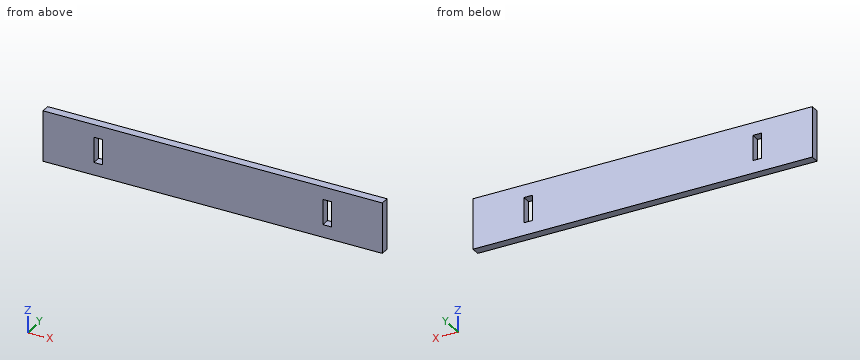
```python
from build123d import *

# Parameters (mm, degrees)
F1_DEPTH = 3.175


with BuildPart() as f1:
    # F0 (on Front) → F1 (new body)
    with BuildSketch(Plane.XZ):
        Polygon((-63.5, 9.525), (-63.5, 0), (-44.45, 0), (-44.45, 4.7625), (-41.275, 4.7625), (-41.275, 0), (0, 0), (41.275, 0), (41.275, 4.7625), (44.45, 4.7625), (44.45, 0), (63.5, 0), (63.5, 9.525), align=None)
        Polygon((-44.45, 0), (-63.5, 0), (-63.5, -9.525), (0, -9.525), (0, 0), (-41.275, 0), (-41.275, -4.7625), (-44.45, -4.7625), align=None)
        Polygon((0, 0), (0, -9.525), (63.5, -9.525), (63.5, 0), (44.45, 0), (44.45, -4.7625), (41.275, -4.7625), (41.275, 0), align=None)
    extrude(amount=F1_DEPTH)


solid = f1.part
```
Can you work these out from the model? Positions are in its coordinate system, mm. Give positions to 0.01 mm unless a question says otherwise; leave off trailing zeros. Loops run counter-clockwise (first coordinate to the right, second up) from the corner with the lowest first, then second, coordinate; pieces in that order, holes last. Notation, with made-up numbers: M 54,-5.5 L 101,-5.5 A8 ccw 101,0.5 Z; hole C 62,82.5 d4. An arc over 180 degrees is marked long. Answer in a Markdown table with one row per item.
1. Suppose I cut it at A-A on z = 0.25. Write out the boundary of the cut face in (x, y) (3 decimals), plus the area to 3 significant figures.
Taken from the geometry:
| item | result |
|---|---|
| outline | M -63.5,-3.175 L -44.45,-3.175 L -44.45,0 L -63.5,0 Z; M -41.275,-3.175 L 41.275,-3.175 L 41.275,0 L -41.275,0 Z; M 44.45,-3.175 L 63.5,-3.175 L 63.5,0 L 44.45,0 Z |
| area | 383 mm² |
2. Suppose I cut it at B-B on y = -2.3. Count the separate pieces of the cut face and the enclosed holes in it, plus the area to 3 significant figures.
Taken from the geometry:
| item | result |
|---|---|
| separate pieces | 1 |
| enclosed holes | 2 |
| area | 2,360 mm² |
3. If I drill on line 1 along X through (y, z) = (-1.45, 3.5) (3 decimals), over which ranges is the centre line in solid material (lowest first)?
Taken from the geometry:
| item | result |
|---|---|
| line 1 | x = -63.5 to -44.45, -41.275 to 41.275, 44.45 to 63.5 |
